Part model, mm, in its own coordinate system. Round coordinates to 2 decimals unless told otherwise and drop trailing zeros. Write each loop counter-clockwise with the first axis right and the second up, starting at its lowest first coordinate (ties: lowest second). Pieces come first, ordered by that corner, then holes. Notation, with made-up numbers: M 64,69.25 L 106,69.25 A33 cw 106,107.25 Z; hole C 11.5,62 d7. An arc over 180 degrees is marked long. Use a Markdown table: item, result. Add a question column.
1) Slice it at A-A on z = 2.5. Write the cut outline in (x, y), plus the area to 3 significant figures.
2) Wall check: probe 1 along X at (y, z) = (18.5, 6.25). Give the ranges that are in metal, low to high.
3) Slice it at B-B on y = -16.5. Write the cut outline in (x, z).
4) Drop flat-ended pins along their axis: P1, Ø3, axis at x = 107, y = -16.5, coming from the -Z side; P2, Ø3, axis at y = 1, z = 3.5, coming from the -X side. Give the stop position or say it passes through.
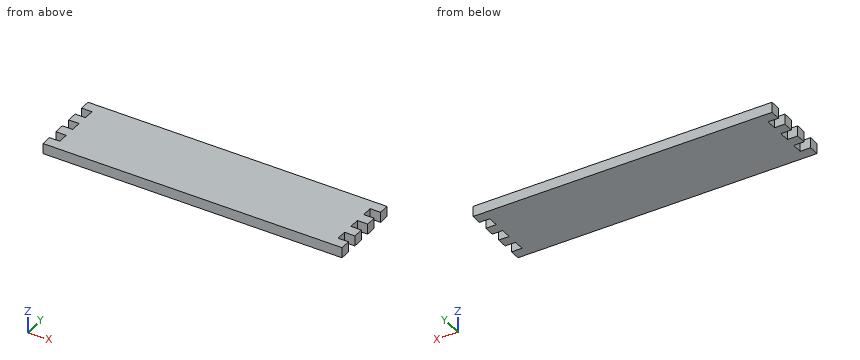
```python
from build123d import *

# Parameters (mm, degrees)
F0_W     = 10
F0_H     = 10
F1_DEPTH = 10


# Not quite as in the source:
# - a feature names something its author has since deleted; it is built from what else it names


with BuildPart() as f1:
    # F0 (on Top) → F1 (new body)
    with BuildSketch(Plane.XY):
        Polygon((131.1653250098, 36.9413525529), (-135.6346749902, 36.9413525529), (-135.6346749902, 26.9413525529), (-135.6346749902, 16.9413525529), (-135.6346749902, 6.9413525529), (-135.6346749902, -3.0586474471), (-135.6346749902, -13.0586474471), (-135.6346749902, -23.0586474471), (-135.6346749902, -33.0586474471), (131.1653250098, -33.0586474471), (131.1653250098, -23.0586474471), (131.1653250098, -13.0586474471), (131.1653250098, -3.0586474471), (131.1653250098, 6.9413525529), (131.1653250098, 16.9413525529), (131.1653250098, 26.9413525529), align=None)
        with Locations((-140.6346749902, 31.9413525529)):
            Rectangle(F0_W, F0_H)
        with Locations((-140.6346749902, 11.9413525529)):
            Rectangle(F0_W, F0_H)
        with Locations((-140.6346749902, -8.0586474471)):
            Rectangle(F0_W, F0_H)
        with Locations((-140.6346749902, -28.0586474471)):
            Rectangle(F0_W, F0_H)
        with Locations((136.1653250098, 31.9413525529)):
            Rectangle(F0_W, F0_H)
        with Locations((136.1653250098, 11.9413525529)):
            Rectangle(F0_W, F0_H)
        with Locations((136.1653250098, -8.0586474471)):
            Rectangle(F0_W, F0_H)
        with Locations((136.1653250098, -28.0586474471)):
            Rectangle(F0_W, F0_H)
    extrude(amount=F1_DEPTH)


solid = f1.part
```
Entries:
| question | item | result |
|---|---|---|
| 1 | outline | M -145.63,-33.06 L 141.17,-33.06 L 141.17,-23.06 L 131.17,-23.06 L 131.17,-13.06 L 141.17,-13.06 L 141.17,-3.06 L 131.17,-3.06 L 131.17,6.94 L 141.17,6.94 L 141.17,16.94 L 131.17,16.94 L 131.17,26.94 L 141.17,26.94 L 141.17,36.94 L -145.63,36.94 L -145.63,26.94 L -135.63,26.94 L -135.63,16.94 L -145.63,16.94 L -145.63,6.94 L -135.63,6.94 L -135.63,-3.06 L -145.63,-3.06 L -145.63,-13.06 L -135.63,-13.06 L -135.63,-23.06 L -145.63,-23.06 Z |
| 1 | area | 19,500 mm^2 |
| 2 | probe 1 | x = -135.63 to 131.17 |
| 3 | outline | M -135.63,0 L 131.17,0 L 131.17,10 L -135.63,10 Z |
| 4 | P1 | stops at z = 0 |
| 4 | P2 | stops at x = -135.63 |
